Autodesk Inventor part; units mm, degrees
ref_plane "YZ Plane" through (0, 0, 0) normal (1, 0, 0) x (0, 1, 0)
ref_plane "XZ Plane" through (0, 0, 0) normal (0, 1, 0) x (-1, 0, 0)
ref_plane "XY Plane" through (0, 0, 0) normal (0, 0, 1) x (1, 0, 0)
ref_plane "Arbeitsebene1" through (0, 0, 0) normal (0, 0, 1) x (1, 0, 0)
sketch "Skizze1" plane through (0, 0, 0) normal (0, 0, 1) x (1, 0, 0)
  circle A0 centre (0, -25) radius 2.5
  circle A1 centre (0, 25) radius 2.5
  line L0 (12.5, -37) -> (12.5, 37)
  line L1 (12.5, 37) -> (-12.5, 37)
  line L2 (-12.5, 37) -> (-12.5, -37)
  line L3 (-12.5, -37) -> (12.5, -37)
  line L4 (0.75, -9.25) -> (-0.75, -9.25)
  line L5 (-0.75, -9.25) -> (-0.75, 9.25)
  line L6 (-0.75, 9.25) -> (0.75, 9.25)
  line L7 (0.75, 9.25) -> (0.75, -9.25)
  circle A2 centre (8.5, -30) radius 1.4
  circle A3 centre (-8.5, -30) radius 1.4
  circle A4 centre (-8.5, 30) radius 1.4
  circle A5 centre (8.5, 30) radius 1.4
  point P0 (0, 0)
extrude "Extrusion1" add sketch "Skizze1" along normal blind 4 contours L3 L2 L1 L0 | L4 L5 L6 L7 | A2 | A3 | A4 | A5
sketch "Skizze2" plane through (0, 0, 0) normal (0, 0, -1) x (-1, 0, 0)
  line L0 (9.25, 9.25) -> (-9.25, 9.25)
  line L1 (9.25, -9.25) -> (9.25, 9.25)
  line L2 (-9.25, -9.25) -> (9.25, -9.25)
  line L3 (-9.25, 9.25) -> (-9.25, -9.25)
  point P0 (0, 0)
extrude "Extrusion2" add sketch "Skizze2" along normal blind 0.3
sketch "Skizze3" plane through (0, 0, -0.3) normal (0, 0, -1) x (-1, 0, 0)
  line L0 (0.75, 7.25) -> (-0.75, 7.25)
  line L1 (0.75, -23.701) -> (0.75, 23.701)
  line L2 (-0.75, 23.701) -> (-0.75, -23.701)
  line L3 (-0.75, -7.25) -> (0.75, -7.25)
  line L4 (0.75, 7.25) -> (-0.75, 7.25)
  line L5 (-0.75, 7.25) -> (-0.75, -7.25)
  line L6 (-0.75, -7.25) -> (0.75, -7.25)
  line L7 (0.75, -7.25) -> (0.75, 7.25)
  point P0 (0, 0)
extrude "Extrusion3" add sketch "Skizze3" along normal blind 0.3
properties part number "40_microfluidic_chip_lightsheet_layer1_negative_mould_lower_v0"
Input: part model. Units: mm. Frame: model coordinates. Coordinates: 2 decimals unless noted, no trailing zeros. Order: outer loops, then holes, each group sorted by start corner. A loop starts at its lowest first (then second) coordinate and runs counter-clockwise, first axis right, second up.
1. Cut plane D-D, the plane y = 26.5. Return loops of the section in (x, z).
Checked values:
outline: (-12.5, 0) - (-2, 0) - (-2, 4) - (-12.5, 4) - close; (2, 0) - (12.5, 0) - (12.5, 4) - (2, 4) - close
2. Cut plane A-A, the plane y = -25. Return loops of the section in (x, z).
Checked values:
outline: (-12.5, 0) - (-2.5, 0) - (-2.5, 4) - (-12.5, 4) - close; (2.5, 0) - (12.5, 0) - (12.5, 4) - (2.5, 4) - close
3. Contact query for flat-ended pins moving along their axis: P1, Ø4.5, axis at x = 0, y = -25, coming from the -Z side; P2, Ø6.5, axis at x = 0, y = 25, coming from the +Z side; P3, Ø1.5, axis at x = -10, y = -12.5, coming from the -Z side. Output: stop coordinate, or through.
Checked values:
P1: passes through
P2: stops at z = 4
P3: stops at z = 0
4. Draft query along X for faces 1 (the cylindrical face through (-0.33, 22.52, 1.97)), 2 (the flat face through (0, 0, -0.6)), 3 (the flat face through (12.5, -1, 2)). Return one class per face: +X half, -X half, draft (parallel to the pull), parting line (faces both ways), or undercut.
Checked values:
face 1: undercut
face 2: draft
face 3: +X half
5. Ray query, line 1 along Y through (x, z) = (0, 2.45); line 2 along Y through (x, z) = (1.75, 2.25); line 3 along Z through (x, y) = (-6.75, -32.5). Return the intervals inside material, ascending.
Checked values:
line 1: y = -37 to -27.5, -22.5 to 22.5, 27.5 to 37
line 2: y = -37 to -26.79, -23.21 to 23.21, 26.79 to 37
line 3: z = 0 to 4
6. Cut plane C-C, the plane x = -6.75. Return loops of the section in (y, z), plus the area to 3 significant figures.
Checked values:
outline: (-37, 0) - (-9.25, 0) - (-9.25, -0.3) - (9.25, -0.3) - (9.25, 0) - (37, 0) - (37, 4) - (-37, 4) - close
area: 302 mm2
7. Cut plane B-B, the plane x = 0. Return loops of the section in (y, z).
Checked values:
outline: (-37, 0) - (-27.5, 0) - (-27.5, 4) - (-37, 4) - close; (-22.5, 0) - (-9.25, 0) - (-9.25, -0.3) - (-7.25, -0.3) - (-7.25, -0.6) - (7.25, -0.6) - (7.25, -0.3) - (9.25, -0.3) - (9.25, 0) - (22.5, 0) - (22.5, 4) - (-22.5, 4) - close; (27.5, 0) - (37, 0) - (37, 4) - (27.5, 4) - close
